Here's how the part is built. I have some questions about the finished solid (model axes, mm). A direction names the side the tool comes from. Round coordinates to 2 decimals unless told otherwise and drop trailing zeros. Write each loop counter-clockwise with the first axis right and the second up, starting at its lowest first coordinate (ties: lowest second). Pieces come first, ordered by that corner, then holes. Notation, with made-up numbers: (36.25, 83) - (72.25, 83) arc R22 cw to (72.25, 118) - close; hole circle Ø8 at (34.25, -18.75). An arc over 180 degrees is marked (long way). Use one line per item in the form item = value. Start each with the question number.
1. I want a section at C-C, the plane y = -28. List the corners of the cut face in (x, z) for me.
2. If I drill on line 1 along X through (y, z) = (-54.5, 7); line 2 along Z through (x, y) = (-24, -85); line 3 along Y through (x, z) = (18, 19), over which ranges is the centre line in solid material (lowest first)?
3. I want a section at A-A, the plane z = 2.25. List the corners of the cut face in (x, y) for me.
4. I want a section at B-B, the plane x = 41.5. List the corners of the cut face in (y, z) for me.
5. We'd pull the mould along X, two halves only. Please class faces 6 (the flat face through (42, -71.752, 15)), 7 (the flat face through (51.737, -34.63, 4.93)), 8 (the cylindrical face through (-31.025, -73.396, 14.93)): +X half, -X half, draft (parallel to the pull), parting line (faces both ways), or undercut.
6. I want a section at D-D, the plane x = -44.5. List the corners of the cut face in (y, z) for me.
7. Which directions (+Z, -Z, +X, -X, +Y, -Y) give clear straight access to the entire face, cutting with the end or side of a thin tool? Please do faces 1 (the cylindrical face through (-31.1, -77.8, 14.9)), 2 (the flat face through (-50.79, -34.11, 4.93)), 3 (the cylindrical face through (24.279, -84.634, 14.93)), 4 (the flat face through (0, -15.697, 5)), 5 (the flat face through (-41, -71.752, 15)).
8. Will these pins go through, and if not, where does the flat tip stop? pin 1 (12 mm diameter, centred on y = -58.5, z = 6, fed in from +X); pin 2 (1 mm diameter, centred on x = -11, y = -82, fed in from -Z); pin 3 (11 mm diameter, centred on x = -41, z = 16.5, fed in from +Y); pin 4 (2 mm diameter, centred on x = 27, z = 9.5, fed in from -Y).
```python
from build123d import *

# Parameters (mm, degrees)
BOSS_EXTRUDE1_DEPTH = 10
SKETCH4_W           = 147.370034426
SKETCH4_H           = 21.427690466
CUT_EXTRUDE1_DEPTH  = 10
SKETCH5_W           = 178.746295464
SKETCH5_H           = 112.332779524
CUT_EXTRUDE2_DEPTH  = 10
BOSS_EXTRUDE2_DEPTH = 10


with BuildPart() as part:
    # Sketch2 → Boss-Extrude1 (new body)
    with BuildSketch(Plane.XY):
        with BuildLine():
            Line((24.926564885, 56.003129771), (45.126564885, -53.996870229))
            ThreePointArc((45.126564885, -53.996870229), (0.426564885, -98.696870229), (-44.273435115, -53.996870229))
            Line((-44.273435115, -53.996870229), (-24.073435115, 56.003129771))
            ThreePointArc((-24.073435115, 56.003129771), (0.426564885, 80.503129771), (24.926564885, 56.003129771))
        make_face()
        with BuildLine():
            ThreePointArc((34.912427768, 56.990682917), (0.426564885, 90.503129771), (-34.059297997, 56.990682917))
            Line((-34.059297997, 56.990682917), (-54.265079147, -53.040798592))
            Line((-54.265079147, -53.040798592), (-44.097865596, -53.040798592))
            Line((-44.097865596, -53.040798592), (-24.073435115, 56.003129771))
            ThreePointArc((-24.073435115, 56.003129771), (0.426564885, 80.503129771), (24.926564885, 56.003129771))
            Line((24.926564885, 56.003129771), (44.950995367, -53.040798592))
            Line((44.950995367, -53.040798592), (55.118208918, -53.040798592))
            Line((55.118208918, -53.040798592), (34.912427768, 56.990682917))
        make_face()
        with BuildLine():
            Line((-44.097865596, -53.040798592), (-54.265079147, -53.040798592))
            ThreePointArc((-54.265079147, -53.040798592), (0.426564885, -108.696870229), (55.118208918, -53.040798592))
            Line((55.118208918, -53.040798592), (44.950995367, -53.040798592))
            Line((44.950995367, -53.040798592), (45.126564885, -53.996870229))
            ThreePointArc((45.126564885, -53.996870229), (0.426564885, -98.696870229), (-44.273435115, -53.996870229))
            Line((-44.273435115, -53.996870229), (-44.097865596, -53.040798592))
        make_face()
    extrude(amount=BOSS_EXTRUDE1_DEPTH)

    # Sketch4 → Cut-Extrude1 (cut)
    with BuildSketch(Plane.XY.offset(10)):
        with Locations((2.831713815, -116.410715462)):
            Rectangle(SKETCH4_W, SKETCH4_H)
    extrude(amount=-CUT_EXTRUDE1_DEPTH, mode=Mode.SUBTRACT)

    # Sketch5 → Cut-Extrude2 (cut)
    with BuildSketch(Plane.XY.offset(10)):
        with Locations((1.072635833, 40.469519533)):
            Rectangle(SKETCH5_W, SKETCH5_H)
    extrude(amount=-CUT_EXTRUDE2_DEPTH, mode=Mode.SUBTRACT)

    # Sketch7 → Boss-Extrude2 (add)
    with BuildSketch(Plane.XY.offset(10)):
        with BuildLine():
            ThreePointArc((18.272585974, -85.111995747), (9.46948112, -88.758361168), (0.022585974, -90.002068509))
            Line((0.022585974, -90.002068509), (0.426564885, -105.696870229))
            Line((0.426564885, -105.696870229), (18.292734033, -105.696870229))
            ThreePointArc((18.292734033, -105.696870229), (39.146778966, -92.634093493), (52.164780298, -71.752068509))
            Line((52.164780298, -71.752068509), (31.632513212, -71.752068509))
            ThreePointArc((31.632513212, -71.752068509), (31.182961311, -72.837382806), (31.029627529, -74.002068509))
            ThreePointArc((31.029627529, -74.002068509), (31.062741779, -74.546982904), (31.161597173, -75.083877552))
            ThreePointArc((31.161597173, -75.083877552), (31.282420431, -75.740082121), (31.322893404, -76.406088604))
            ThreePointArc((31.322893404, -76.406088604), (30.964488909, -78.359033984), (29.935985893, -80.057454127))
            ThreePointArc((29.935985893, -80.057454127), (28.306857221, -81.786339756), (26.577971592, -83.415468427))
            ThreePointArc((26.577971592, -83.415468427), (24.242573732, -84.642622104), (21.604395017, -84.641079707))
            ThreePointArc((21.604395017, -84.641079707), (19.892817757, -84.553395532), (18.272585974, -85.111995747))
        make_face()
        with BuildLine():
            Line((0.426564885, -105.696870229), (0.022585974, -90.002068509))
            ThreePointArc((0.022585974, -90.002068509), (-9.424309172, -88.758361168), (-18.227414026, -85.111995747))
            ThreePointArc((-18.227414026, -85.111995747), (-19.684925655, -84.873628919), (-21.141112037, -85.119962255))
            ThreePointArc((-21.141112037, -85.119962255), (-23.779290752, -85.121504652), (-26.114688612, -83.894350975))
            ThreePointArc((-26.114688612, -83.894350975), (-28.067407493, -82.039534694), (-29.890813945, -80.057454127))
            ThreePointArc((-29.890813945, -80.057454127), (-31.117967622, -77.722056267), (-31.116425225, -75.083877552))
            ThreePointArc((-31.116425225, -75.083877552), (-31.028741049, -73.372300292), (-31.587341264, -71.752068509))
            Line((-31.587341264, -71.752068509), (-51.311650527, -71.752068509))
            ThreePointArc((-51.311650527, -71.752068509), (-38.293649195, -92.634093493), (-17.439604262, -105.696870229))
            Line((-17.439604262, -105.696870229), (0.426564885, -105.696870229))
        make_face()
    extrude(amount=BOSS_EXTRUDE2_DEPTH)


solid = part.part
```
Model answer:
q1.outline = (-49.67, 0) - (50.52, 0) - (50.52, 10) - (-49.67, 10) - close
q2.line_1 = -54.27 to 55.12
q2.line_2 = 0 to 10
q2.line_3 = -105.7 to -85.27
q3.outline = (-54.27, -53.04) arc R54.7 ccw to (-17.44, -105.7) - (18.29, -105.7) arc R54.7 ccw to (55.12, -53.04) - (48.26, -15.7) - (-47.41, -15.7) - close
q4.outline = (-90.12, 0) - (-15.7, 0) - (-15.7, 10) - (-71.75, 10) - (-71.75, 20) - (-90.12, 20) - close
q5.face_6 = draft
q5.face_7 = +X half
q5.face_8 = undercut
q6.outline = (-85.2, 0) - (-15.7, 0) - (-15.7, 10) - (-71.75, 10) - (-71.75, 20) - (-85.2, 20) - close
q7.face_1 = +Z
q7.face_2 = +Z, -Z, -X, +Y
q7.face_3 = +Z, +Y
q7.face_4 = +Z, -Z, +X, -X, +Y
q7.face_5 = +Z, +X, -X, +Y
q8.pin_1 = 55.13
q8.pin_2 = 0
q8.pin_3 = -71.75
q8.pin_4 = -102.35
